The listing builds one solid part. Answer for the finished solid, in the listing's coordinates (mm). A direction names the side the tool comes from. Coordinates: 2 decimals unless noted, no trailing zeros. Order: outer loops, then holes, each group sorted by start corner. A loop starts at its lowest first (then second) coordinate and runs counter-clockwise, first axis right, second up. Notation, with made-up numbers: (-33, 71.5) -> (7, 71.5) arc R24 ccw to (7, 95.5) -> close; hole circle Ø9 at (58.5, -13.5). An arc over 180 degrees is marked (long way). Answer in a Markdown table with one row per item.
```python
from build123d import *

# Parameters (mm, degrees)
SKETCH2_W               = 381
SKETCH2_H               = 1727.2
BOSS_EXTRUDE1_DEPTH     = 18.288
SKETCH3_W               = 18.288
SKETCH3_H               = 76.2
BOSS_EXTRUDE2_DEPTH     = 18.288
LPATTERN1_COUNT         = 5
LPATTERN1_PITCH         = 381
MIRROR1_COPY_1_SKETCH_W = 18.288
MIRROR1_COPY_1_SKETCH_H = 76.2
MIRROR1_COPY_1_DEPTH    = 18.288
MIRROR1_COPY_2_SKETCH_W = 18.288
MIRROR1_COPY_2_SKETCH_H = 76.2
MIRROR1_COPY_2_DEPTH    = 18.288
MIRROR1_COPY_3_SKETCH_W = 18.288
MIRROR1_COPY_3_SKETCH_H = 76.2
MIRROR1_COPY_3_DEPTH    = 18.288
MIRROR1_COPY_4_SKETCH_W = 18.288
MIRROR1_COPY_4_SKETCH_H = 76.2
MIRROR1_COPY_4_DEPTH    = 18.288
CUT_EXTRUDE2_DEPTH      = 1896.363726014
CUT_EXTRUDE4_DEPTH      = 6.35
SKETCH7_R               = 3.175
CUT_EXTRUDE6_DEPTH      = 25.4
SKETCH8_W               = 558.8
SKETCH8_H               = 508
CUT_EXTRUDE7_DEPTH      = 25.4
FILLET1_R               = 50.8
SKETCH10_R              = 3.175
CUT_EXTRUDE8_DEPTH      = 25.4
SKETCH12_R              = 3.175
CUT_EXTRUDE9_DEPTH      = 1896.363726014
SKETCH13_R              = 3.175
CUT_EXTRUDE10_DEPTH     = 1896.363726014


with BuildPart() as part:
    # Sketch2 → Boss-Extrude1 (new body)
    with BuildSketch(Plane.XY):
        with Locations((190.5, 863.6)):
            Rectangle(SKETCH2_W, SKETCH2_H)
    boss_extrude1 = extrude(amount=-BOSS_EXTRUDE1_DEPTH)

    # Sketch3 → Boss-Extrude2 (add)
    with BuildSketch(Plane.XY):
        with Locations((-9.144, 88.9)):
            Rectangle(SKETCH3_W, SKETCH3_H)
    boss_extrude2 = extrude(amount=-BOSS_EXTRUDE2_DEPTH)

    # LPattern1: Boss-Extrude2 ×5
    with Locations(*[(0, i * LPATTERN1_PITCH, 0) for i in range(1, LPATTERN1_COUNT)]):
        add(boss_extrude2)

    # Mirror1: Boss-Extrude1, Boss-Extrude2 across plane
    add(boss_extrude1.mirror(Plane(origin=(381, 0, -18.288), x_dir=(0, 0, 1), z_dir=(1, 0, 0))))
    add(boss_extrude2.mirror(Plane(origin=(381, 0, -18.288), x_dir=(0, 0, 1), z_dir=(1, 0, 0))))

    # Mirror1 copy 1 sketch → Mirror1 copy 1 (add)
    with BuildSketch(Plane(origin=(762, 381, 0), x_dir=(-1, 0, 0), z_dir=(0, 0, 1))):
        with Locations((-9.144, -88.9)):
            Rectangle(MIRROR1_COPY_1_SKETCH_W, MIRROR1_COPY_1_SKETCH_H)
    extrude(amount=-MIRROR1_COPY_1_DEPTH)

    # Mirror1 copy 2 sketch → Mirror1 copy 2 (add)
    with BuildSketch(Plane(origin=(762, 762, 0), x_dir=(-1, 0, 0), z_dir=(0, 0, 1))):
        with Locations((-9.144, -88.9)):
            Rectangle(MIRROR1_COPY_2_SKETCH_W, MIRROR1_COPY_2_SKETCH_H)
    extrude(amount=-MIRROR1_COPY_2_DEPTH)

    # Mirror1 copy 3 sketch → Mirror1 copy 3 (add)
    with BuildSketch(Plane(origin=(762, 1143, 0), x_dir=(-1, 0, 0), z_dir=(0, 0, 1))):
        with Locations((-9.144, -88.9)):
            Rectangle(MIRROR1_COPY_3_SKETCH_W, MIRROR1_COPY_3_SKETCH_H)
    extrude(amount=-MIRROR1_COPY_3_DEPTH)

    # Mirror1 copy 4 sketch → Mirror1 copy 4 (add)
    with BuildSketch(Plane(origin=(762, 1524, 0), x_dir=(-1, 0, 0), z_dir=(0, 0, 1))):
        with Locations((-9.144, -88.9)):
            Rectangle(MIRROR1_COPY_4_SKETCH_W, MIRROR1_COPY_4_SKETCH_H)
    extrude(amount=-MIRROR1_COPY_4_DEPTH)

    # Sketch4 → Cut-Extrude2 (cut, through all)
    with BuildSketch(Plane.XY):
        with BuildLine():
            Line((177.8, 1600.2), (584.2, 1600.2))
            ThreePointArc((584.2, 1600.2), (620.121024484, 1585.321024484), (635, 1549.4))
            Line((635, 1549.4), (635, 889))
            ThreePointArc((635, 889), (620.121024484, 853.078975516), (584.2, 838.2))
            Line((584.2, 838.2), (177.8, 838.2))
            ThreePointArc((177.8, 838.2), (141.878975516, 853.078975516), (127, 889))
            Line((127, 889), (127, 1549.4))
            ThreePointArc((127, 1549.4), (141.878975516, 1585.321024484), (177.8, 1600.2))
        make_face()
    extrude(amount=-CUT_EXTRUDE2_DEPTH, mode=Mode.SUBTRACT)

    # Sketch5 → Cut-Extrude4 (cut)
    with BuildSketch(Plane.XY):
        with BuildLine():
            Line((177.8, 1625.6), (584.2, 1625.6))
            ThreePointArc((584.2, 1625.6), (638.081536726, 1603.281536726), (660.4, 1549.4))
            Line((660.4, 1549.4), (660.4, 889))
            ThreePointArc((660.4, 889), (638.081536726, 835.118463274), (584.2, 812.8))
            Line((584.2, 812.8), (177.8, 812.8))
            ThreePointArc((177.8, 812.8), (123.918463274, 835.118463274), (101.6, 889))
            Line((101.6, 889), (101.6, 1549.4))
            ThreePointArc((101.6, 1549.4), (123.918463274, 1603.281536726), (177.8, 1625.6))
        make_face()
        with BuildLine():
            Line((177.8, 1600.2), (584.2, 1600.2))
            ThreePointArc((584.2, 1600.2), (620.121024484, 1585.321024484), (635, 1549.4))
            Line((635, 1549.4), (635, 889))
            ThreePointArc((635, 889), (620.121024484, 853.078975516), (584.2, 838.2))
            Line((584.2, 838.2), (177.8, 838.2))
            ThreePointArc((177.8, 838.2), (141.878975516, 853.078975516), (127, 889))
            Line((127, 889), (127, 1549.4))
            ThreePointArc((127, 1549.4), (141.878975516, 1585.321024484), (177.8, 1600.2))
        make_face(mode=Mode.SUBTRACT)
    extrude(amount=-CUT_EXTRUDE4_DEPTH, mode=Mode.SUBTRACT)

    # Sketch7 → Cut-Extrude6 (cut)
    with BuildSketch(Plane.XY.offset(-6.35)):
        with Locations((381, 825.5)):
            Circle(SKETCH7_R)
        with Locations((515.62, 825.5)):
            Circle(SKETCH7_R)
        with Locations(Location((246.38, 825.5, 0), (0, 0, 180))):
            Circle(SKETCH7_R)
        with Locations(Location((381, 1612.9, 0), (0, 0, 180))):
            Circle(SKETCH7_R)
        with Locations(Location((114.3, 1219.2, 0), (0, 0, 180))):
            Circle(SKETCH7_R)
        with Locations((515.62, 1612.9)):
            Circle(SKETCH7_R)
        with Locations(Location((246.38, 1612.9, 0), (0, 0, 180))):
            Circle(SKETCH7_R)
        with Locations(Location((114.3, 1353.82, 0), (0, 0, 180))):
            Circle(SKETCH7_R)
        with Locations(Location((114.3, 1488.44, 0), (0, 0, 180))):
            Circle(SKETCH7_R)
        with Locations((114.3, 949.96)):
            Circle(SKETCH7_R)
        with Locations((114.3, 1084.58)):
            Circle(SKETCH7_R)
        with Locations(Location((647.7, 1084.58, 0), (0, 0, 180))):
            Circle(SKETCH7_R)
        with Locations(Location((647.7, 949.96, 0), (0, 0, 180))):
            Circle(SKETCH7_R)
        with Locations((647.7, 1488.44)):
            Circle(SKETCH7_R)
        with Locations((647.7, 1353.82)):
            Circle(SKETCH7_R)
        with Locations((647.7, 1219.2)):
            Circle(SKETCH7_R)
    extrude(amount=-CUT_EXTRUDE6_DEPTH, mode=Mode.SUBTRACT)

    # Sketch8 → Cut-Extrude7 (cut)
    with BuildSketch(Plane.XY):
        with Locations((381, 406.4)):
            Rectangle(SKETCH8_W, SKETCH8_H)
    extrude(amount=-CUT_EXTRUDE7_DEPTH, mode=Mode.SUBTRACT)

    # Fillet1
    fillet1_edges = [part.edges().sort_by_distance(p)[0] for p in [
        (101.6, 152.4, -9.144),
        (101.6, 660.4, -9.144),
        (660.4, 660.4, -9.144),
        (660.4, 152.4, -9.144),
    ]]
    fillet(fillet1_edges, radius=FILLET1_R)

    # Sketch10 → Cut-Extrude8 (cut)
    with BuildSketch(Plane.XY.offset(-6.35)):
        with Locations((131.268636066, 1592.300329375)):
            Circle(SKETCH10_R)
        with Locations(Location((131.268636066, 846.099670625, 0), (0, 0, 180))):
            Circle(SKETCH10_R)
        with Locations((630.731363934, 846.099670625)):
            Circle(SKETCH10_R)
        with Locations(Location((630.731363934, 1592.300329375, 0), (0, 0, 180))):
            Circle(SKETCH10_R)
    extrude(amount=-CUT_EXTRUDE8_DEPTH, mode=Mode.SUBTRACT)

    # Sketch12 → Cut-Extrude9 (cut, through all)
    with BuildSketch(Plane(origin=(0, 0, -18.288), x_dir=(-1, 0, 0), z_dir=(0, 0, -1))):
        with Locations((-177.8, 774.7)):
            Circle(SKETCH12_R)
        with Locations((-279.4, 774.7)):
            Circle(SKETCH12_R)
        with Locations((-381, 774.7)):
            Circle(SKETCH12_R)
        with Locations((-482.6, 774.7)):
            Circle(SKETCH12_R)
        with Locations((-584.2, 774.7)):
            Circle(SKETCH12_R)
        with Locations((-177.8, 19.05)):
            Circle(SKETCH12_R)
        with Locations((-279.4, 19.05)):
            Circle(SKETCH12_R)
        with Locations((-381, 19.05)):
            Circle(SKETCH12_R)
        with Locations((-482.6, 19.05)):
            Circle(SKETCH12_R)
        with Locations((-584.2, 19.05)):
            Circle(SKETCH12_R)
    extrude(amount=-CUT_EXTRUDE9_DEPTH, mode=Mode.SUBTRACT)

    # Sketch13 → Cut-Extrude10 (cut, through all)
    with BuildSketch(Plane(origin=(0, 0, -18.288), x_dir=(-1, 0, 0), z_dir=(0, 0, -1))):
        with Locations((-584.2, 1657.35)):
            Circle(SKETCH13_R)
        with Locations((-482.6, 1657.35)):
            Circle(SKETCH13_R)
        with Locations((-381, 1657.35)):
            Circle(SKETCH13_R)
        with Locations((-279.4, 1657.35)):
            Circle(SKETCH13_R)
        with Locations((-177.8, 1657.35)):
            Circle(SKETCH13_R)
    extrude(amount=-CUT_EXTRUDE10_DEPTH, mode=Mode.SUBTRACT)


solid = part.part
```
(1) Find the intervals of material crossed by line 1 along Y through (x, z) = (246.38, -12) (3 decimals); line 2 along X through (y, z) = (1219.2, -10) (3 decimals); line 3 along Y through (x, z) = (183, -10.5), in increasing order. Write a range as from..to.
Check values:
| item | result |
|---|---|
| line 1 | 0..152.4, 660.4..822.325, 828.675..838.2, 1600.2..1609.725, 1616.075..1727.2 |
| line 2 | -18.288..111.125, 117.475..127, 635..644.525, 650.875..780.288 |
| line 3 | 0..152.4, 660.4..838.2, 1600.2..1727.2 |
(2) A cutting plane is placed at C-C, the plane z = -12.75. Count the separate pieces of the cut face and the enclosed holes in it, then the cut area to 3 significant figures.
Check values:
| item | result |
|---|---|
| separate pieces | 1 |
| enclosed holes | 37 |
| area | 662,000 mm² |
(3) Flat-ended cylindrical pins translate along their axes: pin 1 (5.5 mm diameter, centred on x = 772.5, z = -12, fed in from -Y); pin 2 (8.5 mm diameter, centred on x = 630.73, y = 846.1, fed in from +Z); pin 3 (8 mm diameter, centred on y = 673, z = -11.5, fed in from +X). Find the tip coordinate at first contact, or state that the pin passes through.
Check values:
| item | result |
|---|---|
| pin 1 | y = 50.8 |
| pin 2 | z = -6.35 |
| pin 3 | x = 762 |
(4) A cutting plane is placed at B-B, the plane y = 1122.5. Determine the outline of the cut face in (x, z).
Check values:
| item | result |
|---|---|
| outline | (0, -18.29) -> (127, -18.29) -> (127, -6.35) -> (101.6, -6.35) -> (101.6, 0) -> (0, 0) -> close; (635, -18.29) -> (762, -18.29) -> (762, 0) -> (660.4, 0) -> (660.4, -6.35) -> (635, -6.35) -> close |
(5) A cutting plane is placed at D-D, the plane y = 726. Determine the outline of the cut face in (x, z), then the cut area to 3 significant figures.
Check values:
| item | result |
|---|---|
| outline | (0, -18.29) -> (762, -18.29) -> (762, 0) -> (0, 0) -> close |
| area | 13,900 mm² |
(6) A cutting plane is placed at A-A, the plane x = 355. Determine the outline of the cut face in (y, z), then the cut area to 3 significant figures.
Check values:
| item | result |
|---|---|
| outline | (0, -18.29) -> (152.4, -18.29) -> (152.4, 0) -> (0, 0) -> close; (660.4, -18.29) -> (838.2, -18.29) -> (838.2, -6.35) -> (812.8, -6.35) -> (812.8, 0) -> (660.4, 0) -> close; (1600.2, -18.29) -> (1727.2, -18.29) -> (1727.2, 0) -> (1625.6, 0) -> (1625.6, -6.35) -> (1600.2, -6.35) -> close |
| area | 8,040 mm² |
(7) For a pull along X with two mould halves and no side action, classify faces 1 (the cylindrical face through (637.486, 1603.871, -3.131)), 2 (the flat face through (387, 684, -18.288)), 3 (the cylindrical face through (123.329, 1602.686, -3.131)) as released by +X, released by -X, zero draft, split by the parting line, or undercut.
Check values:
| item | result |
|---|---|
| face 1 | undercut |
| face 2 | zero draft |
| face 3 | undercut |
(8) Which of the six approach directions +Z, -Z, +X, -X, +Y, -Y give full straight-line access (tool end or side, diameter ignored) to faces 4 (the flat face through (651, 1221, -6.35)), 5 (the cylindrical face through (116.086, 645.124, -9.272)), 6 (the flat face through (387, 684, 0))?
Check values:
| item | result |
|---|---|
| face 4 | +Z |
| face 5 | +Z, -Z |
| face 6 | +Z, +X, -X, +Y, -Y |
